Autodesk Inventor part; units mm, degrees
ref_plane "YZ Plane" through (0, 0, 0) normal (1, 0, 0) x (0, 1, 0)
ref_plane "XZ Plane" through (0, 0, 0) normal (0, 1, 0) x (-1, 0, 0)
ref_plane "XY Plane" through (0, 0, 0) normal (0, 0, 1) x (1, 0, 0)
sketch "Sketch1" plane through (0, 0, 0) normal (0, 1, 0) x (-1, 0, 0)
  line L0 (0, 0) -> (35.179, 0)
  line L1 (35.179, 0) -> (35.179, -210.947)
  line L2 (35.179, -210.947) -> (0, -210.947)
  line L3 (0, -210.947) -> (0, 0)
  circle A0 centre (35.179, 0) radius 1.45
  circle A1 centre (0, 0) radius 1.45
  circle A2 centre (35.179, -210.947) radius 1.45
  line L4 (-6.35, 6.35) -> (41.529, 6.35)
  line L5 (41.529, 6.35) -> (41.529, -217.297)
  line L6 (41.529, -217.297) -> (-6.35, -217.297)
  line L7 (-6.35, -217.297) -> (-6.35, 6.35)
  line L8 (-6.35, 6.35) -> (41.529, -217.297) construction
  line L9 (41.529, 6.35) -> (-6.35, -217.297) construction
  line L10 (28.829, -204.597) -> (41.529, -204.597)
  line L11 (41.529, -204.597) -> (41.529, -217.297)
  line L12 (41.529, -217.297) -> (28.829, -217.297)
  line L13 (28.829, -217.297) -> (28.829, -204.597)
  line L14 (28.829, -204.597) -> (41.529, -217.297) construction
  line L15 (41.529, -204.597) -> (28.829, -217.297) construction
  line L16 (-9.525, 9.525) -> (44.704, 9.525)
  line L17 (44.704, 9.525) -> (44.704, -220.472)
  line L18 (44.704, -220.472) -> (-9.525, -220.472)
  line L19 (-9.525, -220.472) -> (-9.525, 9.525)
  line L20 (-9.525, 9.525) -> (44.704, -220.472) construction
  line L21 (44.704, 9.525) -> (-9.525, -220.472) construction
  point P0 (17.5895, -105.4735)
  point P1 (17.5895, -105.4735)
  dimension "d0" = 35.179
  dimension "d1" = 210.947
  dimension "d2" = 2.9
  dimension "d3" = 2.9
  dimension "d4" = 2.9
  dimension "d6" = 12.7
  dimension "d7" = 12.7
  dimension "d8" = 3.175
  dimension "d9" = 3.175
extrude "Extrusion1" add sketch "Sketch1" along normal blind 3.175 contours A1 L3 L2 L13 L6 L7 L4 L5 L10 L1 A0 L0 | L0 A0 L1 L10 L13 L2 L3 A1 | L13 L10 L1 A2 L2 | L2 A2 L1 L10 L5 L6 L13 | L16 L17 L18 L19
extrude "Extrusion2" add sketch "Sketch1" along normal blind 22.225
sketch "Sketch2" plane through (0, 3.175, 0) normal (0, 1, 0) x (1, 0, 0)
  circle A0 centre (-35.1446, 0) radius 3.175
  circle A1 centre (0, 0) radius 3.175
  circle A2 centre (-35.179, 0) radius 1.45
  circle A3 centre (0, 0) radius 1.45
  circle A4 centre (-35.179, 210.947) radius 1.45
  circle A5 centre (-35.179, 210.947) radius 3.175
  point P0 (0, 210.947)
  dimension "d14" = 6.35
  dimension "d15" = 6.35
  dimension "d20" = 6.35
extrude "Extrusion3" add sketch "Sketch2" along normal blind 6.35
extrude "Extrusion4" add sketch "Sketch1" along normal blind 3.175 contours L3 A1 L0 | L0 A1 L3 | A0 L1 L0 | L0 L1 A0 | A2 L1 L2 | L2 L1 A2
sketch "Sketch3" plane through (0, 22.225, 0) normal (0, 1, 0) x (1, 0, 0)
  circle A0 centre (-25.011, 12.319) radius 6.5
  circle A1 centre (-25.011, 50.292) radius 6.5
  circle A2 centre (-25.011, 64.516) radius 6.5
  circle A3 centre (-25.011, 102.489) radius 6.5
  circle A4 centre (-25.011, 116.713) radius 6.5
  circle A5 centre (-25.011, 154.686) radius 6.5
  circle A6 centre (-25.011, 168.91) radius 6.5
  circle A7 centre (-25.011, 206.883) radius 6.5
  line L0 (-9.707, 199.896) -> (-9.707, 209.896)
  line L1 (-9.707, 209.896) -> (2.293, 209.896)
  line L2 (2.293, 209.896) -> (2.293, 199.896)
  line L3 (2.293, 199.896) -> (-9.707, 199.896)
  line L4 (-9.707, 177.003) -> (2.293, 177.003)
  line L5 (-9.707, 167.003) -> (-9.707, 177.003)
  line L6 (2.293, 167.003) -> (-9.707, 167.003)
  line L7 (2.293, 177.003) -> (2.293, 167.003)
  line L8 (2.293, 157.699) -> (2.293, 147.699)
  line L9 (-9.707, 157.699) -> (2.293, 157.699)
  line L10 (2.293, 147.699) -> (-9.707, 147.699)
  line L11 (-9.707, 147.699) -> (-9.707, 157.699)
  line L12 (-9.707, 124.806) -> (2.293, 124.806)
  line L13 (-9.707, 114.806) -> (-9.707, 124.806)
  line L14 (2.293, 114.806) -> (-9.707, 114.806)
  line L15 (2.293, 124.806) -> (2.293, 114.806)
  line L16 (-9.707, 105.502) -> (2.293, 105.502)
  line L17 (2.293, 105.502) -> (2.293, 95.502)
  line L18 (-9.707, 95.502) -> (-9.707, 105.502)
  line L19 (2.293, 95.502) -> (-9.707, 95.502)
  line L20 (-9.707, 72.609) -> (2.293, 72.609)
  line L21 (-9.707, 62.609) -> (-9.707, 72.609)
  line L22 (2.293, 62.609) -> (-9.707, 62.609)
  line L23 (2.293, 72.609) -> (2.293, 62.609)
  line L24 (-9.707, 53.305) -> (2.293, 53.305)
  line L25 (-9.707, 43.305) -> (-9.707, 53.305)
  line L26 (2.293, 43.305) -> (-9.707, 43.305)
  line L27 (2.293, 53.305) -> (2.293, 43.305)
  line L28 (-9.707, 20.412) -> (2.293, 20.412)
  line L29 (2.293, 20.412) -> (2.293, 10.412)
  line L30 (2.293, 10.412) -> (-9.707, 10.412)
  line L31 (-9.707, 10.412) -> (-9.707, 20.412)
  line L32 (-17.686, -1.671) -> (-20.286, -1.671)
  line L33 (-23.811, 2.214) -> (-23.811, 0.214)
  line L34 (-14.161, 2.214) -> (-14.161, 0.214)
  line L35 (-18.511, 3.894) -> (-17.511, 3.894)
  line L36 (-20.461, 3.894) -> (-19.461, 3.894)
  line L37 (-35.859, 30.096) -> (-35.859, 20.096)
  line L38 (-35.859, 42.669) -> (-35.859, 32.669)
  line L39 (-35.859, 82.293) -> (-35.859, 72.293)
  line L40 (-35.859, 94.866) -> (-35.859, 84.866)
  line L41 (-35.859, 134.49) -> (-35.859, 124.49)
  line L42 (-35.859, 147.063) -> (-35.859, 137.063)
  line L43 (-35.859, 186.687) -> (-35.859, 176.687)
  line L44 (-35.859, 199.26) -> (-35.859, 189.26)
  line L45 (-17.0795, 187.3678) -> (-17.0795, 189.3599)
  line L46 (-13.5395, 185.2639) -> (-17.0795, 185.2639)
  line L47 (-17.0795, 191.4639) -> (-13.5395, 191.4639)
  line L48 (-13.5395, 191.4639) -> (-13.5395, 185.2639)
  line L49 (-13.5395, 139.2668) -> (-13.5395, 133.0668)
  line L50 (-17.0795, 139.2668) -> (-13.5395, 139.2668)
  line L51 (-17.0795, 135.1708) -> (-17.0795, 137.1629)
  line L52 (-13.5395, 133.0668) -> (-17.0795, 133.0668)
  line L53 (-13.5395, 87.0699) -> (-13.5395, 80.8699)
  line L54 (-13.5395, 80.8699) -> (-17.0795, 80.8699)
  line L55 (-17.0795, 87.0699) -> (-13.5395, 87.0699)
  line L56 (-17.0795, 82.9738) -> (-17.0795, 84.9659)
  line L57 (-17.0795, 30.7768) -> (-17.0795, 32.7689)
  line L58 (-13.5395, 28.6728) -> (-17.0795, 28.6728)
  line L59 (-17.0795, 34.8728) -> (-13.5395, 34.8728)
  line L60 (-13.5395, 34.8728) -> (-13.5395, 28.6728)
  line L61 (3.1921, 139.1709) -> (3.1921, 133.1709)
  line L62 (3.1921, 86.9739) -> (3.1921, 80.9739)
  line L63 (3.1921, 34.7769) -> (3.1921, 28.7769)
  line L64 (3.1921, 191.3679) -> (3.1921, 185.3679)
  circle A8 centre (-35.179, 0) radius 1.702
  circle A9 centre (0, 0) radius 1.702
  circle A10 centre (-35.179, 210.947) radius 1.702
  line L65 (9.525, 220.472) -> (-44.704, 220.472)
  line L66 (-44.704, 220.472) -> (-44.704, -9.525)
  line L67 (-44.704, -9.525) -> (9.525, -9.525)
  line L68 (9.525, -9.525) -> (9.525, 220.472)
  line L69 (6.35, -6.35) -> (-41.529, -6.35)
  line L70 (-41.529, -6.35) -> (-41.529, 217.297)
  line L71 (-41.529, 217.297) -> (6.35, 217.297)
  line L72 (6.35, 217.297) -> (6.35, -6.35)
  line L73 (9.525, -9.525) -> (9.525, 220.472)
  line L74 (6.35, 20.412) -> (9.525, 20.412)
  line L75 (9.525, 20.412) -> (9.525, 43.305)
  line L76 (9.525, 43.305) -> (6.35, 43.305)
  line L77 (6.35, 43.305) -> (6.35, 20.412)
  line L78 (6.35, 217.297) -> (6.35, -6.35)
  line L79 (6.35, 72.609) -> (9.525, 72.609)
  line L80 (9.525, 72.609) -> (9.525, 95.502)
  line L81 (9.525, 95.502) -> (6.35, 95.502)
  line L82 (6.35, 95.502) -> (6.35, 72.609)
  line L83 (6.35, 124.806) -> (9.525, 124.806)
  line L84 (9.525, 124.806) -> (9.525, 147.699)
  line L85 (9.525, 147.699) -> (6.35, 147.699)
  line L86 (6.35, 147.699) -> (6.35, 124.806)
  line L87 (6.35, 177.003) -> (9.525, 177.003)
  line L88 (9.525, 177.003) -> (9.525, 199.896)
  line L89 (9.525, 199.896) -> (6.35, 199.896)
  line L90 (6.35, 199.896) -> (6.35, 177.003)
  line L91 (-41.529, 217.297) -> (-41.529, -6.35)
  line L92 (-44.704, 220.472) -> (-44.704, -9.525)
  line L93 (-41.529, 20.412) -> (-44.704, 20.412)
  line L94 (-44.704, 20.412) -> (-44.704, 43.305)
  line L95 (-44.704, 43.305) -> (-41.529, 43.305)
  line L96 (-41.529, 43.305) -> (-41.529, 20.412)
  line L97 (-41.529, 72.293) -> (-44.704, 72.293)
  line L98 (-44.704, 72.293) -> (-44.704, 95.502)
  line L99 (-44.704, 95.502) -> (-41.529, 95.502)
  line L100 (-41.529, 95.502) -> (-41.529, 72.293)
  line L101 (-41.529, 124.806) -> (-44.704, 124.806)
  line L102 (-44.704, 124.806) -> (-44.704, 147.699)
  line L103 (-44.704, 147.699) -> (-41.529, 147.699)
  line L104 (-41.529, 147.699) -> (-41.529, 124.806)
  line L105 (-41.529, 177.003) -> (-44.704, 177.003)
  line L106 (-44.704, 177.003) -> (-44.704, 199.896)
  line L107 (-44.704, 199.896) -> (-41.529, 199.896)
  line L108 (-41.529, 199.896) -> (-41.529, 177.003)
  point P0 (0, 0)
extrude "Extrusion5" cut sketch "Sketch3" against normal blind 12.7 contours L107 L70 L105 L66 | L103 L70 L101 L66 | L99 L70 L97 L66 | L95 L70 L93 L66
extrude "Extrusion6" cut sketch "Sketch3" against normal up to surface (19.05 mm away) contours L68 L87 L72 L89 | L68 L83 L72 L85 | L68 L79 L72 L81 | L68 L74 L72 L76
fillet "Fillet1" radius 3.175 16 edges at (7.9375, 3.175, -20.412) (7.9375, 3.175, -43.305) (7.9375, 3.175, -72.609) (7.9375, 3.175, -95.502) (7.9375, 3.175, -124.806) (7.9375, 3.175, -147.699) (7.9375, 3.175, -199.896) (7.9375, 3.175, -177.003) (-43.1165, 9.525, -20.412) (-43.1165, 9.525, -43.305) (-43.1165, 9.525, -95.502) (-43.1165, 9.525, -147.699) (-43.1165, 9.525, -199.896) (-43.1165, 9.525, -72.293) (-43.1165, 9.525, -124.806) (-43.1165, 9.525, -177.003)
fillet "Fillet2" radius 3.175 4 edges at (9.525, 11.1125, 9.525) (9.525, 11.1125, -220.472) (-44.704, 11.1125, -220.472) (-44.704, 11.1125, 9.525)
properties part number "Box"
For this review, take the finished solid that the model builds, in its own axes (mm). A direction names the side the tool comes from. Round coordinates to 2 decimals unless told otherwise and drop trailing zeros. Write each loop counter-clockwise with the first axis right and the second up, starting at its lowest first coordinate (ties: lowest second). Pieces come first, ordered by that corner, then holes. Notation, with made-up numbers: M 43.25,79 L 79.25,79 A6 cw 79.25,83 Z; hole C 34,36.25 d8. An arc over 180 degrees is marked long. Write item = value, one per line. Start each with the question number.
(1) We need section C-C (y = 16.75). Give the number of separate pieces and of enclosed holes in the cut face, then the cut area to 3 significant figures.
(2) For faces 4 (the face through (-37, 9.525, -211)), 5 (the face through (-17, 11, 9.525)), list the 3-axis set-ups (+Z, -Z, +X, -X, +Y, -Y) from which the entire face can be reached by the end or side of a thin tool; tool diameter is ignored.
(3) The part is to be moulded in two halves that separate along Z. For faces 1 (the face through (6.35, 13, -9)), 2 (the face through (-18, 11, -220.472)), 3 (the face through (-17, 22.225, 7)), say which applies: +Z half, -Z half, draft (parallel to the pull), parting line (faces both ways), or undercut.
(4) We need section B-B (z = -9). Give the boundary of the cut face in (x, y) (3 decimals), then the cut area to 3 significant figures.
(5) For line 1 along X through (y, z) = (7.5, 0) (3 decimals); line 2 along Z through (x, y) = (-26.5, 19.75) (3 decimals); line 3 along X through (y, z) = (21.75, -70) (3 decimals), list the stretches that pass through material, from the lowest coordinate up.
(6) We need section A-A (x = -16). Give the boundary of the cut face in (y, z) (3 decimals).
(7) Clearance check with flat-ended pins moving along their axes: pin 1 Ø3.5 at (x, y) = (-44, 15) entering from -Z; pin 2 Ø3.5 at (x, y) = (-43.5, 18) entering from +Z; pin 3 Ø3.5 at (x, z) = (-42.5, -32.5) entering from +Y (3 decimals). State where each tip first meets the part, or that it passes through.
Results found:
q1.separate_pieces = 8
q1.enclosed_holes = 0
q1.area = 1,170 mm²
q2.face_4 = +Y
q2.face_5 = +Z, +X, -X, +Y, -Y
q3.face_1 = undercut
q3.face_2 = -Z half
q3.face_3 = draft
q4.outline = M -44.704,0 L 9.525,0 L 9.525,22.225 L 6.35,22.225 L 6.35,3.175 L -41.529,3.175 L -41.529,22.225 L -44.704,22.225 Z
q4.area = 293 mm²
q5.line_1 = -44.704 to -41.529, -38.32 to -36.629, -33.729 to -31.97, -3.175 to -1.45, 1.45 to 3.175, 6.35 to 9.525
q5.line_2 = -220.472 to -217.297, 6.35 to 9.525
q5.line_3 = -44.704 to -41.529, 6.35 to 9.525
q6.outline = M 0,-220.472 L 22.225,-220.472 L 22.225,-217.297 L 3.175,-217.297 L 3.175,6.35 L 22.225,6.35 L 22.225,9.525 L 0,9.525 Z
q7.pin_1 = -220.39
q7.pin_2 = 9.52
q7.pin_3 = 9.525
